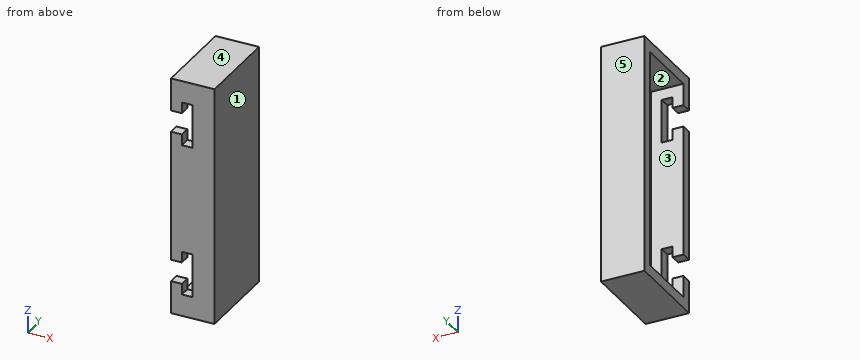
from build123d import *

# Parameters (mm, degrees)
SKETCH1_W           = 25.4
SKETCH1_H           = 139.7
BOSS_EXTRUDE1_DEPTH = 6.35
SKETCH3_W           = 25.4
SKETCH3_H           = 6.35
BOSS_EXTRUDE2_DEPTH = 38.1
BOSS_EXTRUDE3_DEPTH = 6.35
CUT_EXTRUDE2_DEPTH  = 84.521209881
SKETCH8_W           = 12.7
SKETCH8_H           = 139.7
CUT_EXTRUDE3_DEPTH  = 84.521209881
SKETCH9_W           = 6.35
SKETCH9_H           = 127
BOSS_EXTRUDE4_DEPTH = 38.1
SKETCH10_W          = 25.4
SKETCH10_H          = 139.7
BOSS_EXTRUDE5_DEPTH = 6.35


with BuildPart() as part:
    # Sketch1 → Boss-Extrude1 (new body)
    with BuildSketch(Plane(origin=(0, 0, 0), x_dir=(1, 0, 0), z_dir=(0, 1, 0))):
        Rectangle(SKETCH1_W, SKETCH1_H)
    extrude(amount=BOSS_EXTRUDE1_DEPTH)

    # Sketch3 → Boss-Extrude2 (add)
    with BuildSketch(Plane(origin=(0, 6.35, 0), x_dir=(1, 0, 0), z_dir=(0, 1, 0))):
        with Locations((0, 66.675)):
            Rectangle(SKETCH3_W, SKETCH3_H)
        with Locations((0, -66.675)):
            Rectangle(SKETCH3_W, SKETCH3_H)
    extrude(amount=BOSS_EXTRUDE2_DEPTH)

    # Sketch6 → Boss-Extrude3 (add)
    with BuildSketch(Plane(origin=(0, 6.35, 0), x_dir=(1, 0, 0), z_dir=(0, 1, 0))):
        Polygon((12.7, 50.8), (19.05, 50.8), (19.05, 57.15), (25.4, 57.15), (25.4, 31.75), (19.05, 31.75), (19.05, 38.1), (12.7, 38.1), align=None)
    boss_extrude3 = extrude(amount=-BOSS_EXTRUDE3_DEPTH)

    # Sketch7 → Cut-Extrude2 (cut, through all)
    with BuildSketch(Plane(origin=(0, 6.35, 0), x_dir=(1, 0, 0), z_dir=(0, 1, 0))):
        Polygon((-12.7, 50.8), (-6.35, 50.8), (-6.35, 57.15), (0, 57.15), (0, 31.75), (-6.35, 31.75), (-6.35, 38.1), (-12.7, 38.1), align=None)
    cut_extrude2 = extrude(amount=-CUT_EXTRUDE2_DEPTH, mode=Mode.SUBTRACT)

    # Mirror1: Boss-Extrude3, Cut-Extrude2 across plane
    add(boss_extrude3.mirror(Plane.XY))
    add(cut_extrude2.mirror(Plane.XY), mode=Mode.SUBTRACT)

    # Sketch8 → Cut-Extrude3 (cut, through all)
    with BuildSketch(Plane(origin=(0, 6.35, 0), x_dir=(1, 0, 0), z_dir=(0, 1, 0))):
        with Locations((19.05, 0)):
            Rectangle(SKETCH8_W, SKETCH8_H)
    extrude(amount=-CUT_EXTRUDE3_DEPTH, mode=Mode.SUBTRACT)

    # Sketch9 → Boss-Extrude4 (add)
    with BuildSketch(Plane(origin=(0, 6.35, 0), x_dir=(1, 0, 0), z_dir=(0, 1, 0))):
        with Locations((9.525, 0)):
            Rectangle(SKETCH9_W, SKETCH9_H)
    extrude(amount=BOSS_EXTRUDE4_DEPTH)

    # Sketch10 → Boss-Extrude5 (add)
    with BuildSketch(Plane(origin=(0, 44.45, 0), x_dir=(1, 0, 0), z_dir=(0, 1, 0))):
        Rectangle(SKETCH10_W, SKETCH10_H)
    extrude(amount=BOSS_EXTRUDE5_DEPTH)


solid = part.part
Part model, mm, in its own coordinate system. Face numbers are marked on the shaded views. A direction names the side the tool comes from. Coordinates: 2 decimals unless noted, no trailing zeros. Write each loop counter-clockwise with the first axis right and the second up, starting at its lowest first coordinate (ties: lowest second). Pieces come first, ordered by that corner, then holes. Notation, with made-up numbers: M 57.25,62 L 81.25,62 A17 cw 81.25,93 Z; hole C -24.75,39 d2. An arc over 180 degrees is marked long. Return JSON: item names as keys, results as strings.
1. Flat gauge pins, fed straight in: pin 1 Ø3 at (y, z) = (3.5, 43) entering from -X; pin 2 Ø5 at (y, z) = (11, 48.5) entering from -X. Where does each tip first touch, or does it go through?
Determined:
{"pin 1": "x = 0", "pin 2": "x = 6.35"}
2. Saw through at C-C, the plane z = 8. Write the cut outline in (x, y).
Determined:
{"outline": "M -12.7,0 L 12.7,0 L 12.7,50.8 L -12.7,50.8 L -12.7,44.45 L 6.35,44.45 L 6.35,6.35 L -12.7,6.35 Z"}
3. Saw through at D-D, the plane x = 1.5. Write the cut outline in (y, z), then the cut area to 3 significant figures.
Determined:
{"outline": "M 0,-69.85 L 50.8,-69.85 L 50.8,69.85 L 0,69.85 Z; hole M 6.35,-63.5 L 44.45,-63.5 L 44.45,63.5 L 6.35,63.5 Z", "area": "2,260 mm²"}
4. Saw through at B-B, the plane z = -53.5. Write the cut outline in (x, y), then the cut area to 3 significant figures.
Determined:
{"outline": "M -12.7,0 L -6.35,0 L -6.35,6.35 L -12.7,6.35 Z; M -12.7,44.45 L 6.35,44.45 L 6.35,6.35 L 0,6.35 L 0,0 L 12.7,0 L 12.7,50.8 L -12.7,50.8 Z", "area": "524 mm²"}
5. Probe L1, parallel to Z at x = -4.25, y = 3; L2, parallel to Y at x = -6.5, z = 1.5; L3, parallel to Z at x = -5, y = 26.5. List the from-to ranges inside material, lowest first.
Determined:
{"L1": "-69.85 to -57.15, -31.75 to 31.75, 57.15 to 69.85", "L2": "0 to 6.35, 44.45 to 50.8", "L3": "-69.85 to -63.5, 63.5 to 69.85"}
6. 3-axis set-ups, long thin cutter, end or side, ignore diameter. For the marked faces 1 and 2: which of +Z, -Z, +X, -X, +Y, -Y reach the whole face in a straight line?
Determined:
{"face 1": "+Z, -Z, +X, +Y, -Y", "face 2": "-X"}
7. Saw through at A-A, the plane x = -4.5. Write the cut outline in (y, z).
Determined:
{"outline": "M 0,-69.85 L 50.8,-69.85 L 50.8,69.85 L 0,69.85 L 0,57.15 L 6.35,57.15 L 6.35,63.5 L 44.45,63.5 L 44.45,-63.5 L 6.35,-63.5 L 6.35,-57.15 L 0,-57.15 Z; M 0,-31.75 L 6.35,-31.75 L 6.35,31.75 L 0,31.75 Z"}
8. Pull direction Y, two halves, no side cores. Call the marked faces 3, 4 and 5: pulls with the +Y half, pulls with the -Y half, needs draft (parallel to the pull), parting line crosses it, or undercut.
Determined:
{"face 3": "undercut", "face 4": "needs draft", "face 5": "pulls with the +Y half"}
